from build123d import *

# Parameters (mm, degrees)
F0_R     = 11.2
F1_DEPTH = 7


# Not quite as in the source:
# - ends of sketch curves that miss each other by under 0.0002 mm in the source are joined


with BuildPart() as f1:
    # F0 (on Top) → F1 (new body)
    with BuildSketch(Plane.XY):
        with BuildLine():
            ThreePointArc((-8.6004e-06, -13.2), (-13.2, 0), (-8.6004e-06, 13.2))
            Line((-8.6004e-06, 13.2), (-29.4360226951, 13.1999579737))
            ThreePointArc((-29.4360226951, 13.1999579737), (-42.6692934144, 0.0318031051), (-29.4996289049, -13.1999652303))
            ThreePointArc((-29.4996289049, -13.1999652303), (-29.4693403268, -13.2), (-29.4390517487, -13.1999652698))
            Line((-29.4390517487, -13.1999652698), (-8.6004e-06, -13.2))
        make_face()
        with Locations((-29.4693317264, 0)):
            Circle(F0_R, mode=Mode.SUBTRACT)
        with BuildLine():
            ThreePointArc((-8.6004e-06, 13.2), (9.333806471, 9.3338125524), (13.2, 0))
            ThreePointArc((13.2, 0), (9.333806471, -9.3338125524), (-8.6004e-06, -13.2))
            Line((-8.6004e-06, -13.2), (29.4658418158, -13.200003649))
            ThreePointArc((29.4658418158, -13.200003649), (42.6658504162, -3.649e-06), (29.4658418158, 13.199996351))
            Line((29.4658418158, 13.199996351), (-8.6004e-06, 13.2))
        make_face()
        with Locations((29.4658504162, -3.649e-06)):
            Circle(F0_R, mode=Mode.SUBTRACT)
        with BuildLine():
            ThreePointArc((-8.6004e-06, -13.2), (9.333806471, -9.3338125524), (13.2, 0))
            ThreePointArc((13.2, 0), (9.333806471, 9.3338125524), (-8.6004e-06, 13.2))
            ThreePointArc((-8.6004e-06, 13.2), (-13.2, 0), (-8.6004e-06, -13.2))
        make_face()
        Circle(F0_R, mode=Mode.SUBTRACT)
    extrude(amount=F1_DEPTH)


solid = f1.part
Could you check a few things on this model? Use its own coordinates, in mm. Give positions to 0.01 mm unless a question says otherwise; leave off trailing zeros. Order: outer loops, then holes, each group sorted by start corner. A loop starts at its lowest first (then second) coordinate and runs counter-clockwise, first axis right, second up. Notation, with made-up numbers: (26.25, -36) -> (53.25, -36) arc R28 ccw to (53.25, -4) -> close; hole circle Ø4 at (-31, 0). An arc over 180 degrees is marked (long way). Return JSON: item names as keys, results as strings.
1. Imagine slicing it at C-C on y = -7. List the corners of the cut face in (x, z) for me.
Answer list:
{"outline": "(-40.66, 0) -> (-38.21, 0) -> (-38.21, 7) -> (-40.66, 7) -> close; (-20.73, 0) -> (-8.74, 0) -> (-8.74, 7) -> (-20.73, 7) -> close; (8.74, 0) -> (20.72, 0) -> (20.72, 7) -> (8.74, 7) -> close; (38.21, 0) -> (40.66, 0) -> (40.66, 7) -> (38.21, 7) -> close"}
2. Imagine slicing it at A-A on y = -3.5. List the corners of the cut face in (x, z) for me.
Answer list:
{"outline": "(-42.2, 0) -> (-40.11, 0) -> (-40.11, 7) -> (-42.2, 7) -> close; (-18.83, 0) -> (-10.64, 0) -> (-10.64, 7) -> (-18.83, 7) -> close; (10.64, 0) -> (18.83, 0) -> (18.83, 7) -> (10.64, 7) -> close; (40.1, 0) -> (42.19, 0) -> (42.19, 7) -> (40.1, 7) -> close"}
3. I need wall thicknesses on line 1 (X direction, y = -6.25, z = 1.75); line 2 (Y direction, x = 0, z = 2); line 3 (X direction, y = -6, z = 3.75). Which ranges of each line are inside material? Lowest first, please. Write a range as from..to.
Answer list:
{"line 1": "x = -41.1..-38.76, -20.18..-9.29, 9.29..20.17, 38.76..41.09", "line 2": "y = -13.2..-11.2, 11.2..13.2", "line 3": "x = -41.23..-38.93, -20.01..-9.46, 9.46..20.01, 38.92..41.22"}
4. Thinking about a two-plate mould opening in Y: for faces 1 (the cylindrical face through (42.663, -0.29, 3.451)), 2 (the flat face through (-10, -6, 7)), 3 (the cylindrical face through (-40.66, 0.49, 3.45)), which applies, pulls with the +Y half, pulls with the -Y half, needs draft (parallel to the pull), parting line crosses it, or undercut?
Answer list:
{"face 1": "parting line crosses it", "face 2": "needs draft", "face 3": "undercut"}
5. Imagine slicing it at B-B on z = 4.5. List the corners of the cut face in (x, y) for me, then the cut area to 3 significant figures.
Answer list:
{"outline": "(-29.5, -13.2) arc R13.2 ccw to (-29.44, -13.2) -> (0, -13.2) -> (29.47, -13.2) arc R13.2 ccw to (29.47, 13.2) -> (0, 13.2) -> (-29.44, 13.2) arc R13.2 ccw to start; hole circle Ø22.4 at (-29.47, 0); hole circle Ø22.4 at (0, 0); hole circle Ø22.4 at (29.47, 0)", "area": "921 mm2"}
